Input: dimensioned drawing with shaded views. Units: mm. Origin: part minimum x, y, z. A direction names the side the tool comes from. Round coordinates to 2 decimals unless told otherwise and drop trailing zeros. Write each loop counter-clockwise with the first axis right and the second up, starting at its lowest first coordinate (ties: lowest second). Pieces come first, ordered by that corner, then holes. Notation, with made-up numbers: (42.5, 57.5) -> (57.5, 57.5) arc R16 ccw to (57.5, 68.5) -> close; hole circle Ø2 at (-35.5, 79.5). An arc over 180 degrees is marked (long way). One line per item, written item: value. Start each with the question number.
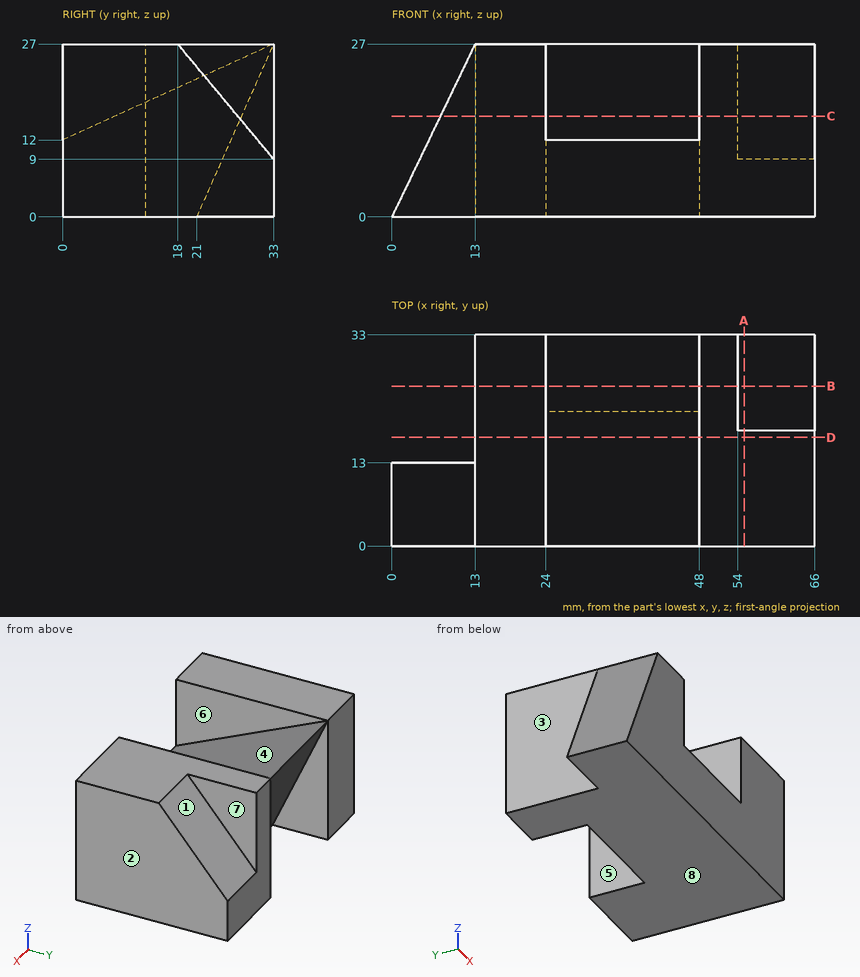
(1) Line query: probe 1 along X at (y, z) = (16.5, 22.75); probe 2 along X at (y, z) = (31.5, 24.75); probe 3 along X at (y, z) = (21, 8.75). Output: solid intervals per line, ascending.
(2) Section query D-D (y = 17). Output: boundary loops of the cut face in (x, z).
(3) Set-up query: the marked faces 1, 2, 3, 4 and 5. Return all of +Z, -Z, +X, -X, +Y, -Y with unobstructed straight access to the full face (end or side cutting, diameter ignored); none if empty.
(4) Section query C-C (z = 15.75). Output: boundary loops of the cut face in (x, y) (3 decimals).
(5) Pin query (flat end, axial travel): pin 1 (10 mm diameter, centred on y = 23, z = 19.5, fed in from -X); pin 2 (1 mm diameter, centred on x = 7.5, z = 10.5, fed in from +Y); pin 3 (8 mm diameter, centred on y = 5, z = 6.5, fed in from -X). Return the tip coordinate at first contact, or that it passes through.
(6) Pull-direction query (X, two-part tool) for the marked faces 6, 7 and 8; classes: pulls with the +X half, pulls with the -X half, needs draft (parallel to the pull), parting line crosses it, or undercut.
(7) Section query A-A (x = 55). Output: boundary loops of the cut face in (y, z), and give its area (3 significant figures).
(8) Section query B-B (y = 25). Output: boundary loops of the cut face in (x, z), and give its area (3 significant figures).
Results list:
1. probe 1: x = 13 to 24, 48 to 66
1. probe 2: x = 13 to 54
1. probe 3: x = 13 to 66
2. outline: (13, 0) -> (66, 0) -> (66, 27) -> (48, 27) -> (48, 19.73) -> (24, 19.73) -> (24, 27) -> (13, 27) -> close
3. face 1: +Z, +X, +Y
3. face 2: +Z, -Z, +X, +Y, -Y
3. face 3: +Z, -Z, -X, +Y
3. face 4: +Z, -Y
3. face 5: -Z, +Y
4. outline: (7.583, 0) -> (24, 0) -> (24, 8.25) -> (48, 8.25) -> (48, 0) -> (66, 0) -> (66, 27.375) -> (54, 27.375) -> (54, 33) -> (48, 33) -> (48, 28) -> (24, 28) -> (24, 33) -> (13, 33) -> (13, 13) -> (7.583, 13) -> close
5. pin 1: stops at x = 13
5. pin 2: stops at y = 13
5. pin 3: stops at x = 1.2
6. face 6: undercut
6. face 7: pulls with the +X half
6. face 8: needs draft
7. outline: (0, 0) -> (33, 0) -> (33, 9) -> (18, 27) -> (0, 27) -> close
7. area: 756 mm^2
8. outline: (13, 0) -> (24, 0) -> (24, 9) -> (48, 9) -> (48, 0) -> (66, 0) -> (66, 18.6) -> (54, 18.6) -> (54, 27) -> (48, 27) -> (48, 23.36) -> (24, 23.36) -> (24, 27) -> (13, 27) -> close
8. area: 1,030 mm^2
